The model under review builds one solid part; all positions refer to its coordinate system, in mm. Coordinates: 2 decimals unless noted, no trailing zeros. Order: outer loops, then holes, each group sorted by start corner. A loop starts at its lowest first (then second) coordinate and runs counter-clockwise, first axis right, second up. Notation, with made-up numbers: (87, 2.25) - (95, 2.25) arc R18 cw to (95, 35.25) - close; hole circle Ø7 at (27.25, 30). An arc over 180 degrees is marked (long way). Answer in a Markdown table with one row per item.
```python
from build123d import *

# Parameters (mm, degrees)
F1_DEPTH = 25.4


with BuildPart() as f1:
    # F0 (on Front) → F1 (new body)
    with BuildSketch(Plane.XZ):
        with BuildLine():
            ThreePointArc((-14.4099858393, -36.15015585), (-9.6174010791, -74.0035828929), (22.5965727608, -53.5558275878))
            ThreePointArc((22.5965727608, -53.5558275878), (20.3675773267, -43.7697714683), (14.1203409545, -35.9143686951))
            ThreePointArc((14.1203409545, -35.9143686951), (-0.1867416275, -30.9600264713), (-14.4099858393, -36.15015585))
        make_face()
        with BuildLine():
            ThreePointArc((-14.4099858393, -36.15015585), (-0.1867416275, -30.9600264713), (14.1203409545, -35.9143686951))
            ThreePointArc((14.1203409545, -35.9143686951), (14.7921035223, -29.4911375194), (12.7136237721, -23.3764759904))
            ThreePointArc((12.7136237721, -23.3764759904), (10.1115297439, -20.1661301682), (6.7352958132, -17.7832205863))
            ThreePointArc((6.7352958132, -17.7832205863), (-0.0550758769, -16.1010168), (-6.8734396529, -17.6659042354))
            ThreePointArc((-6.8734396529, -17.6659042354), (-9.8053911529, -19.5704448334), (-12.2196112726, -22.0993093418))
            ThreePointArc((-12.2196112726, -22.0993093418), (-15.0762108242, -28.8501475286), (-14.4099858393, -36.15015585))
        make_face()
        with BuildLine():
            ThreePointArc((-6.8734396529, -17.6659042354), (-0.0550758769, -16.1010168), (6.7352958132, -17.7832205863))
            ThreePointArc((6.7352958132, -17.7832205863), (0.0906184951, 0.7995784888), (-6.8734396529, -17.6659042354))
        make_face()
    extrude(amount=F1_DEPTH)


solid = f1.part
```
Item 1: We need section A-A, the plane x = -8. Write out the cut boundary in (y, z) (3 decimals).
Check values:
| item | result |
|---|---|
| outline | (-25.4, -74.689) - (0, -74.689) - (0, -18.285) - (-25.4, -18.285) - close; (-25.4, -16.532) - (0, -16.532) - (0, -2.893) - (-25.4, -2.893) - close |
Item 2: Clearance check with flat-ended pins moving along their axes: pin 1 Ø3 at (x, y) = (7.5, -5) entering from +Z; pin 2 Ø3 at (x, z) = (-16, -35.5) entering from +Y; pin 3 Ø3 at (y, z) = (-7.5, -59) entering from +X; pin 4 Ø5 at (y, z) = (-9.5, -44.5) entering from -X. State where each tip first meets the part, or that it passes through.
Check values:
| item | result |
|---|---|
| pin 1 | z = -1.08 |
| pin 2 | y = 0 |
| pin 3 | x = 22.25 |
| pin 4 | x = -21.62 |
Item 3: To check wall thickness, follow line 1 (Z direction, x = -7, y = -15.25); line 2 (Z direction, x = 9, y = -23.5); line 3 (X direction, y = -3, z = -33.5). State the ranges of each line that lie inside material, in increasing order. Write a range as from..to.
Check values:
| item | result |
|---|---|
| line 1 | -75.04..-17.73, -17.55..-1.87 |
| line 2 | -74.28..-19.22, -15.14..-4.28 |
| line 3 | -15.08..14.71 |
Item 4: We need section C-C, the plane z = -20.5. Write out the cut boundary in (x, y).
Check values:
| item | result |
|---|---|
| outline | (-10.83, -25.4) - (10.46, -25.4) - (10.46, 0) - (-10.83, 0) - close |
Item 5: Mouldability with a two-part tool opening along Z and no side actions: class faces 1 (the face through (0, 0, -46)), 2 (the face through (0.45, -12.52, 0.79)) as +Z half, -Z half, draft (parallel to the pull), parting line (faces both ways), or undercut.
Check values:
| item | result |
|---|---|
| face 1 | draft |
| face 2 | undercut |
Item 6: We need section B-B, the plane y = -15.75. Write out the cut boundary in (x, z) (3 decimals), then the cut area to 3 significant figures.
Check values:
| item | result |
|---|---|
| outline | (-14.41, -36.15) arc R22.597 ccw (long way) to (14.12, -35.914) arc R15.071 ccw to (6.735, -17.783) arc R10.512 ccw (long way) to (-6.873, -17.666) arc R15.071 ccw to start |
| area | 2,310 mm^2 |
Item 7: We need section D-D, the plane x = -19. Write out the cut boundary in (y, z).
Check values:
| item | result |
|---|---|
| outline | (-25.4, -65.79) - (0, -65.79) - (0, -41.32) - (-25.4, -41.32) - close |
